Design review of the part shown in the three views and the two pictorial views. Dimensions are in mm from the part's minimum x, y and z. A direction names the side the tool comes from. Give positions to 0.01 mm unless a question says otherwise; leave off trailing zeros. Loops run counter-clockwise (first coordinate to the right, second up) from the corner with the lowest first, then second, coordinate; pieces in that order, holes last. Notation, with made-up numbers: (17, 12) - (66, 12) arc R12 ccw to (66, 19) - close; hole circle Ø6 at (-24.75, -36). An arc over 180 degrees is marked (long way). Answer in a Markdown table with one row per item.
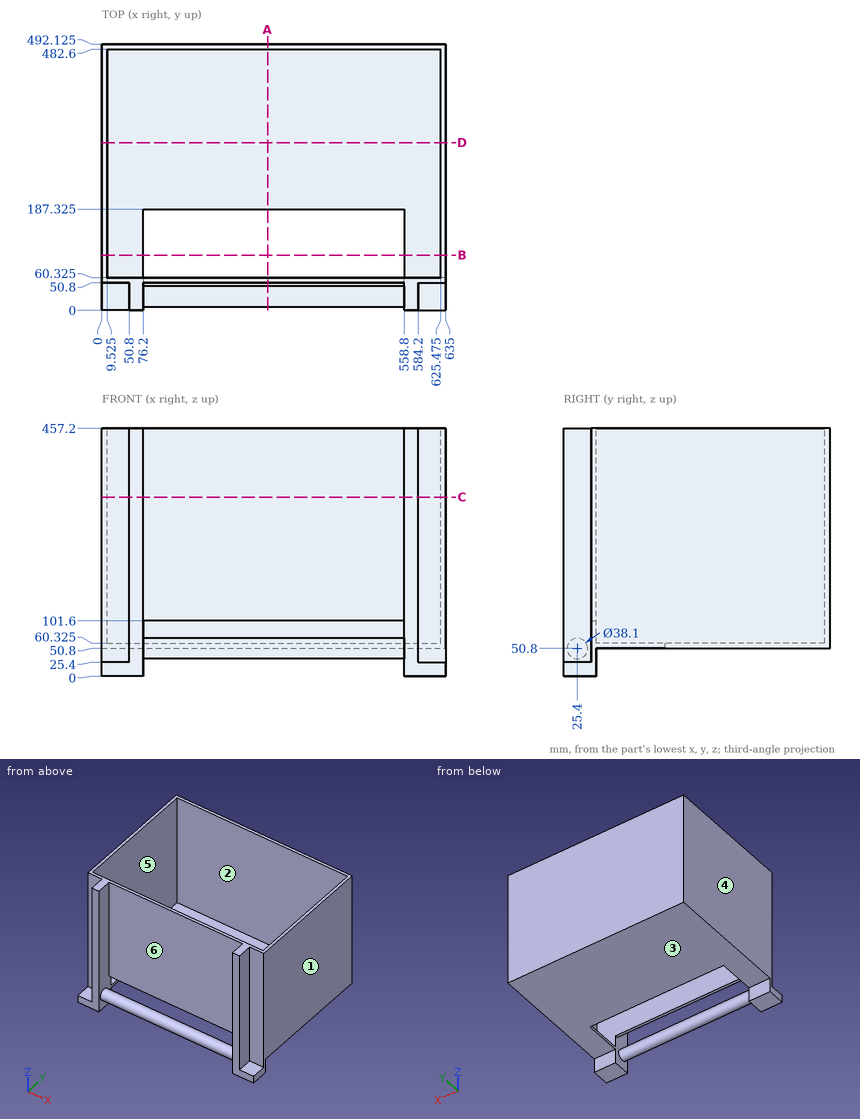
1. We need section C-C, the plane z = 330.5. Give the boundary of the cut face in (x, y) (3 decimals).
Values:
| item | result |
|---|---|
| outline | (0, 50.8) - (50.8, 50.8) - (50.8, 0) - (76.2, 0) - (76.2, 50.8) - (558.8, 50.8) - (558.8, 0) - (584.2, 0) - (584.2, 50.8) - (635, 50.8) - (635, 492.125) - (0, 492.125) - close; hole (9.525, 60.325) - (625.475, 60.325) - (625.475, 482.6) - (9.525, 482.6) - close |
2. We need section A-A, the plane x = 306. Give the boundary of the cut face in (y, z) (3 decimals), and give its area (3 significant figures).
Values:
| item | result |
|---|---|
| outline | circle Ø38.1 at (25.4, 50.8); (50.8, 101.6) - (60.325, 101.6) - (60.325, 457.2) - (50.8, 457.2) - close; (187.325, 50.8) - (492.125, 50.8) - (492.125, 457.2) - (482.6, 457.2) - (482.6, 60.325) - (187.325, 60.325) - close |
| area | 11,200 mm^2 |
3. Wall thickness on line 1 (Y direction, x = 471.5, z = 416) (3 decimals); line 2 (X direction, y = 347, z = 95) (3 decimals); line 3 (X direction, y = 30, z = 140): over which ranges is each line inside the solid? List them lowest first. Write a range as [from, to].
Values:
| item | result |
|---|---|
| line 1 | y = [50.8, 60.325], [482.6, 492.125] |
| line 2 | x = [0, 9.525], [625.475, 635] |
| line 3 | x = [50.8, 76.2], [558.8, 584.2] |
4. We need section D-D, the plane y = 310. Give the boundary of the cut face in (x, z) (3 decimals).
Values:
| item | result |
|---|---|
| outline | (0, 50.8) - (635, 50.8) - (635, 457.2) - (625.475, 457.2) - (625.475, 60.325) - (9.525, 60.325) - (9.525, 457.2) - (0, 457.2) - close |
5. Clearance check with flat-ended pins moving along their axes: pin 1 (1.5 mm diameter, centred on x = 205, z = 359.5, fed in from -Y); pin 2 (3 mm diameter, centred on x = 80, y = 393.5, fed in from +Z) (3 decimals); pin 3 (10.5 mm diameter, centred on x = 234, z = 56, fed in from -Y). State where each tip first meets the part, or that it passes through.
Values:
| item | result |
|---|---|
| pin 1 | stops at y = 50.8 |
| pin 2 | stops at z = 60.325 |
| pin 3 | stops at y = 6.35 |
6. We need section B-B, the plane y = 102. Give the boundary of the cut face in (x, z) (3 decimals).
Values:
| item | result |
|---|---|
| outline | (0, 50.8) - (76.2, 50.8) - (76.2, 60.325) - (9.525, 60.325) - (9.525, 457.2) - (0, 457.2) - close; (558.8, 50.8) - (635, 50.8) - (635, 457.2) - (625.475, 457.2) - (625.475, 60.325) - (558.8, 60.325) - close |
7. Mouldability with a two-part tool opening along Y and no side actions: class the marked faces 4, 5 and 6 as released by +Y, released by -Y, zero draft, split by the parting line, or undercut.
Values:
| item | result |
|---|---|
| face 4 | zero draft |
| face 5 | undercut |
| face 6 | released by -Y |
8. For the marked faces 1, 2 and 3, list the 3-axis set-ups (+Z, -Z, +X, -X, +Y, -Y) from which the entire face can be reached by the end or side of a thin tool; tool diameter is ignored.
Values:
| item | result |
|---|---|
| face 1 | +Z, -Z, +X, +Y, -Y |
| face 2 | +Z |
| face 3 | -Z, +X, -X, +Y |
